Geometry check sheet. Reference: the model listing, model coordinates, mm. Face numbers are marked on the shaded views. A direction names the side the tool comes from. Give positions to 0.01 mm unless a question says otherwise; leave off trailing zeros. Write each loop counter-clockwise with the first axis right and the second up, starting at its lowest first coordinate (ties: lowest second). Pieces come first, ordered by that corner, then holes. Notation, with made-up numbers: (-30.75, -10) -> (4.25, -10) arc R21 cw to (4.25, 26) -> close; hole circle Ø2 at (45.25, 50.25). An arc over 180 degrees is marked (long way). Use a Markdown table: item, result. Add a question column.
from build123d import *

# Parameters (mm, degrees)
SKETCH_1_R               = 0.5
EXTRUDE_1_DEPTH          = 4
CUT_EXTRUDE_1_DEPTH      = 8.679442038
CUT_EXTRUDE_1_DEPTH_BACK = 8.679442038


with BuildPart() as part:
    # 草图1 → 凸台-拉伸1 (new body)
    with BuildSketch(Plane.XY):
        with BuildLine():
            Line((-1.244261308, -4.563724383), (-1.244261308, 5.436275617))
            ThreePointArc((-1.244261308, 5.436275617), (-0.244261308, 6.436275617), (0.755738692, 5.436275617))
            Line((0.755738692, 5.436275617), (0.755738692, -4.563724383))
            Line((0.755738692, -4.563724383), (-1.244261308, -4.563724383))
        make_face()
        with Locations((-0.244261308, 5.436275617)):
            Circle(SKETCH_1_R, mode=Mode.SUBTRACT)
        with Locations((-0.244261308, 0.436275617)):
            Circle(SKETCH_1_R, mode=Mode.SUBTRACT)
    extrude(amount=EXTRUDE_1_DEPTH)

    # 草图4 → 切除-拉伸1 (cut, two sides: drawn at the far end of the back side and taken through both)
    with BuildSketch(Plane(origin=(0, 0, 0), x_dir=(0, 0, -1), z_dir=(1, 0, 0)).offset(-CUT_EXTRUDE_1_DEPTH_BACK)):
        Polygon((-2.875, 39.17528395), (-2.875, 6.436275617), (-2.875, 4.436275617), (-1.125, 4.436275617), (-1.125, 6.436275617), (-1.125, 39.17528395), (-1.125, 104.653300618), (-2.875, 104.653300618), align=None)
    extrude(amount=CUT_EXTRUDE_1_DEPTH + CUT_EXTRUDE_1_DEPTH_BACK, mode=Mode.SUBTRACT)


solid = part.part
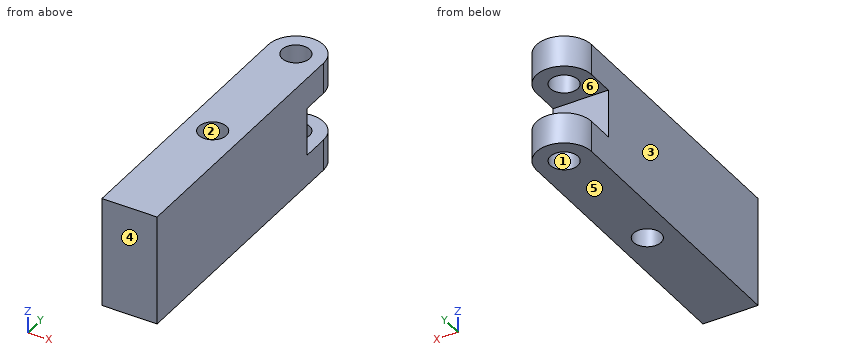
1) Sectioned sample at B-B, the plane z = 2.05. Enter the section's corners in (x, y), and give its area (3 significant figures).
2) Draft check along Y on the marked faces 1, 2, 3 and 4. Enter one of: +Y half, -Y half, draft (parallel to the pull), parting line (faces both ways), or undercut.
3) Sectioned sample at A-A, the plane x = -0.25. Enter the section's corners in (y, z) (3 decimals), and give its area (3 significant figures).
4) Material ranges on probe 1 along Z at (x, y) = (0.15, 6.25) (3 decimals); probe 2 along Y at (x, z) = (-0.4, 0.7); probe 3 along Y at (x, z) = (-0.2, 1.45), recorded low to high. Write a range as [from, to].
5) Sectioned sample at C-C, the plane x = 0.5. Enter the section's corners in (y, z) (3 decimals).
6) Tool access check on the marked faces 5 and 6. Record the directions out of +Z, -Z, +X, -X, +Y, -Y that give a thin tool (end or side, any length) a straight path to the whole face; none if there is none.
7) Sectioned sample at D-D, the plane z = 3.55. Enter the section's corners in (x, y), and give its area (3 significant figures).
Check values:
| question | item | result |
|---|---|---|
| 1 | outline | (-1.24, -4.56) -> (0.76, -4.56) -> (0.76, 4.44) -> (-1.24, 4.44) -> close; hole circle Ø1 at (-0.24, 0.44) |
| 1 | area | 17.2 mm² |
| 2 | face 1 | undercut |
| 2 | face 2 | undercut |
| 2 | face 3 | draft |
| 2 | face 4 | -Y half |
| 3 | outline | (-4.564, 0) -> (-0.064, 0) -> (-0.064, 4) -> (-4.564, 4) -> close; (0.936, 0) -> (4.936, 0) -> (4.936, 1.125) -> (4.436, 1.125) -> (4.436, 2.875) -> (4.936, 2.875) -> (4.936, 4) -> (0.936, 4) -> close; (5.936, 0) -> (6.436, 0) -> (6.436, 1.125) -> (5.936, 1.125) -> close; (5.936, 2.875) -> (6.436, 2.875) -> (6.436, 4) -> (5.936, 4) -> close |
| 3 | area | 34.3 mm² |
| 4 | probe 1 | [0, 1.125], [2.875, 4] |
| 4 | probe 2 | [-4.56, -0.04], [0.91, 4.96], [5.91, 6.42] |
| 4 | probe 3 | [-4.56, -0.06], [0.93, 4.44] |
| 5 | outline | (-4.564, 0) -> (6.104, 0) -> (6.104, 1.125) -> (4.436, 1.125) -> (4.436, 2.875) -> (6.104, 2.875) -> (6.104, 4) -> (-4.564, 4) -> close |
| 6 | face 5 | -Z, +X, -X, +Y, -Y |
| 6 | face 6 | +X, -X, +Y |
| 7 | outline | (-1.24, -4.56) -> (0.76, -4.56) -> (0.76, 5.44) arc R1 ccw to (-1.24, 5.44) -> close; hole circle Ø1 at (-0.24, 0.44); hole circle Ø1 at (-0.24, 5.44) |
| 7 | area | 20.0 mm² |
